Design review of the part built by this model. Coordinates are the model's own, in mm. Face numbers are marked on the shaded views. A direction names the side the tool comes from. Give positions to 0.01 mm unless a question says otherwise; leave off trailing zeros. Write each loop counter-clockwise with the first axis right and the second up, starting at its lowest first coordinate (ties: lowest second). Pieces come first, ordered by that corner, then holes. Notation, with made-up numbers: (73, -8.75) -> (93, -8.75) arc R21 ccw to (93, 16.25) -> close; hole circle Ø6 at (51, 75). An arc over 180 degrees is marked (long way). Put each result on its own line as item: value. Start each with the question number.
from build123d import *

# Parameters (mm, degrees)
SKETCH1_W           = 12
SKETCH1_H           = 12
SKETCH1_W_2         = 5
SKETCH1_H_2         = 5
BOSS_EXTRUDE1_DEPTH = 2.5
SKETCH2_W           = 5
SKETCH2_H           = 5
BOSS_EXTRUDE2_DEPTH = 3.2
SKETCH3_R           = 1.1
CUT_EXTRUDE1_DEPTH  = 20.454819454
FILLET1_R           = 2.5
CUT_EXTRUDE2_DEPTH  = 20.454819454


with BuildPart() as part:
    # Sketch1 → Boss-Extrude1 (new body)
    with BuildSketch(Plane(origin=(0, 0, 0), x_dir=(1, 0, 0), z_dir=(0, 1, 0))):
        Polygon((-6, -10), (-6, 2), (-6, 10), (-11, 10), (-11, -10), align=None)
        with Locations((0, -4)):
            Rectangle(SKETCH1_W, SKETCH1_H)
        Polygon((6, 10), (6, 2), (6, -10), (11, -10), (11, 10), align=None)
        with Locations((8.5, 12.5)):
            Rectangle(SKETCH1_W_2, SKETCH1_H_2)
        with Locations((-8.5, 12.5)):
            Rectangle(SKETCH1_W_2, SKETCH1_H_2)
        Polygon((11, -10), (11, -15), (-11, -15), (-11, -10), (-6, -10), (6, -10), align=None)
    extrude(amount=BOSS_EXTRUDE1_DEPTH)

    # Sketch2 → Boss-Extrude2 (add)
    with BuildSketch(Plane.XZ):
        with Locations((-8.5, -12.5)):
            Rectangle(SKETCH2_W, SKETCH2_H)
        with Locations((-8.5, 12.5)):
            Rectangle(SKETCH2_W, SKETCH2_H)
        with Locations((8.5, -12.5)):
            Rectangle(SKETCH2_W, SKETCH2_H)
        with Locations((8.5, 12.5)):
            Rectangle(SKETCH2_W, SKETCH2_H)
    extrude(amount=BOSS_EXTRUDE2_DEPTH)

    # Sketch3 → Cut-Extrude1 (cut, through all)
    with BuildSketch(Plane(origin=(0, 2.5, 0), x_dir=(1, 0, 0), z_dir=(0, 1, 0))):
        with Locations(Location((-8.5, 12.5, 0), (0, 0, 270))):
            Circle(SKETCH3_R)
        with Locations(Location((-8.5, -12.5, 0), (0, 0, 90))):
            Circle(SKETCH3_R)
        with Locations(Location((8.5, -12.5, 0), (0, 0, 270))):
            Circle(SKETCH3_R)
        with Locations(Location((8.5, 12.5, 0), (0, 0, 90))):
            Circle(SKETCH3_R)
    extrude(amount=-CUT_EXTRUDE1_DEPTH, mode=Mode.SUBTRACT)

    # Fillet1
    fillet1_edges = [part.edges().sort_by_distance(p)[0] for p in [
        (-11, -1.6, -10),
        (6, -1.6, -10),
        (6, -1.6, 10),
        (11, -1.6, -10),
        (-6, -1.6, -10),
        (-11, -1.6, 10),
        (-6, -1.6, 10),
        (11, -1.6, 10),
        (11, -0.35, 15),
        (-6, -1.6, 15),
        (6, -1.6, 15),
        (-11, -0.35, 15),
        (-11, -0.35, -15),
        (-6, -0.35, -15),
        (11, -0.35, -15),
        (6, -0.35, -15),
        (6, 1.25, -2),
        (-6, 1.25, -2),
    ]]
    fillet(fillet1_edges, radius=FILLET1_R - 0.0001)  # a hair under: the kernel refuses the full size

    # Sketch4 → Cut-Extrude2 (cut, through all)
    with BuildSketch(Plane(origin=(0, 2.5, 0), x_dir=(1, 0, 0), z_dir=(0, 1, 0))):
        with BuildLine():
            Line((-3.5, -2), (3.5, -2))
            ThreePointArc((3.5, -2), (5.267766953, -2.732233047), (6, -4.5))
            Line((6, -4.5), (6, -5.5))
            ThreePointArc((6, -5.5), (5.267766953, -7.267766953), (3.5, -8))
            Line((3.5, -8), (-3.5, -8))
            ThreePointArc((-3.5, -8), (-5.267766953, -7.267766953), (-6, -5.5))
            Line((-6, -5.5), (-6, -4.5))
            ThreePointArc((-6, -4.5), (-5.267766953, -2.732233047), (-3.5, -2))
        make_face()
    extrude(amount=-CUT_EXTRUDE2_DEPTH, mode=Mode.SUBTRACT)


solid = part.part
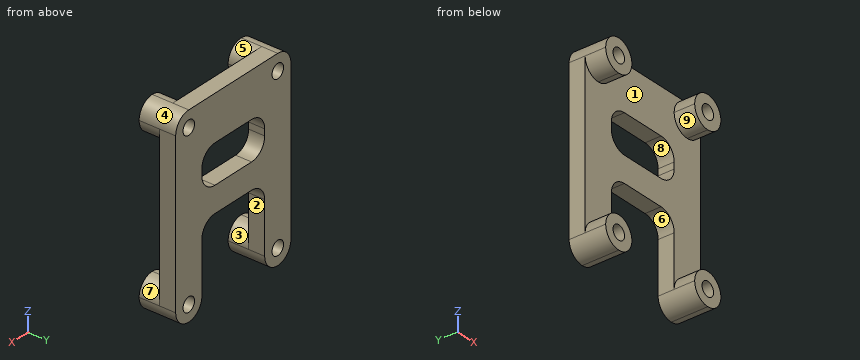
Q1. Take a section at A-A on x = -1.25. Give the boundary of the cut face in (y, z), then the cut area to 3 significant figures.
Q2. Take a section at B-B on z = -9. Give the boundary of the cut face in (x, y), then the cut area to 3 significant figures.
Q3. Take a section at C-C on y = 1.25. State how many separate pieces and enclosed holes the cut face has, then the cut area to 3 significant figures.
Q4. To check wall thickness, follow probe 1 along X at (y, z) = (1.3, 12.5); probe 2 along X at (y, z) = (0, -12.5); probe 3 along X at (y, z) = (0.35, -7.5). State the ranges of each line that lie inside material, in increasing order. Write a range as from..to.
Q5. For pin 1 (12 mm diameter, centred on x = -5, z = -12, fed in from +Y); pin 2 (2 mm diameter, centred on x = 1.5, y = 1, fed in from -Z); pin 3 (3 mm diameter, centred on x = 6, z = -3, fed in from -Y); pin 4 (1 mm diameter, centred on x = 3.5, y = 1, fed in from -Z), all flat-tipped, find the tip position at first contact; note any pin that passes through.
Q6. Mouldability with a two-part tool opening along Z and no side actions: class the marked faces 1, 2, 3 and 4 as +Z half, -Z half, draft (parallel to the pull), parting line (faces both ways), or undercut.
Q7. Machinability: for the marked faces 5, 6, 7, 8 and 9, which of the approach directions +Z, -Z, +X, -X, +Y, -Y give a long, thin tool a straight path to every point of the face, cutting with its end or side? Answer none if there is none.
Result:
1. outline: (0, -2) -> (2.5, -2) -> (2.5, 2) -> (0, 2) -> close; (0, 8) -> (2.5, 8) -> (2.5, 15) -> (0, 15) -> close
1. area: 27.5 mm^2
2. outline: (-11, 0) -> (-6, 0) -> (-6, 2.5) -> (-11, 2.5) -> close; (6, 0) -> (11, 0) -> (11, 2.5) -> (6, 2.5) -> close
2. area: 25.0 mm^2
3. separate pieces: 1
3. enclosed holes: 5
3. area: 417 mm^2
4. probe 1: x = -11..-9.6, -7.4..7.4, 9.6..11
4. probe 2: x = -11..-9.6, -7.4..-6, 6..7.4, 9.6..11
4. probe 3: x = -11..-6, 6..11
5. pin 1: stops at y = 2.5
5. pin 2: stops at z = -2
5. pin 3: stops at y = 0
5. pin 4: stops at z = -2.05
6. face 1: undercut
6. face 2: draft
6. face 3: undercut
6. face 4: +Z half
7. face 5: +Z, -Y
7. face 6: -Z, +Y, -Y
7. face 7: +X, -Y
7. face 8: +Y, -Y
7. face 9: -Y
